from build123d import *

# Parameters (mm, degrees)
SKETCH_1_R      = 1.5
EXTRUDE_2_DEPTH = 24
SKETCH_3_R      = 0.5
EXTRUDE_3_DEPTH = 3.1
FILLET_1_R      = 0.5
SKETCH_4_R      = 3
EXTRUDE_4_DEPTH = 24


with BuildPart() as part:
    # ｽｹｯﾁ1 → ﾎﾞｽ - 押し出し2 (new body)
    with BuildSketch(Plane(origin=(0, 0, 0), x_dir=(1, 0, 0), z_dir=(0, 1, 0))):
        Circle(SKETCH_1_R)
    extrude(amount=EXTRUDE_2_DEPTH)

    # ｽｹｯﾁ3 → ﾎﾞｽ - 押し出し3 (add)
    with BuildSketch(Plane.XZ):
        Circle(SKETCH_3_R)
    extrude(amount=EXTRUDE_3_DEPTH)

    # ﾌｨﾚｯﾄ1
    fillet_1_edges = [part.edges().sort_by_distance(p)[0] for p in [
        (-0.5, -3.1, 0),
    ]]
    fillet(fillet_1_edges, radius=FILLET_1_R)

    # ｽｹｯﾁ4 → ﾎﾞｽ - 押し出し4 (add)
    with BuildSketch(Plane(origin=(0, 24, 0), x_dir=(1, 0, 0), z_dir=(0, 1, 0))):
        Circle(SKETCH_4_R)
    extrude(amount=-EXTRUDE_4_DEPTH)


solid = part.part
Build history of the part. All positions in model axes, mm. A direction names the side the tool comes from. Round coordinates to 2 decimals unless told otherwise and drop trailing zeros. Write each loop counter-clockwise with the first axis right and the second up, starting at its lowest first coordinate (ties: lowest second). Pieces come first, ordered by that corner, then holes. Notation, with made-up numbers: (-14, 2) - (7, 2) arc R19 cw to (7, 15) - close; hole circle Ø11 at (51, -22.5). An arc over 180 degrees is marked (long way). Use CSV: the item, a comma, the result in double quotes.
(1) Band-saw the part on A-A (z = 0). Write the cut outline in (x, y).
Response:
outline,"(-3, 0) - (-0.5, 0) - (-0.5, -2.6) arc R0.5 ccw to (0.5, -2.6) - (0.5, 0) - (3, 0) - (3, 24) - (-3, 24) - close"
(2) Band-saw the part on C-C (y = 16.75). Write the cut outline in (x, z).
Response:
outline,"circle Ø6 at (0, 0)"
(3) 3-axis set-ups, long thin cutter, end or side, ignore diameter. For faces 1 (the cylindrical face through (-3, 12, 0)), 2 (the cylindrical face through (-0.108, -1.282, -0.488)): which of +Z, -Z, +X, -X, +Y, -Y reach the whole face in a straight line?
Response:
face 1,"+Y, -Y"
face 2,"-Y"
(4) Band-saw the part on D-D (x = 2.25). Write the cut outline in (y, z), plus the area to 3 significant figures.
Response:
outline,"(0, -1.98) - (24, -1.98) - (24, 1.98) - (0, 1.98) - close"
area,"95.2 mm²"
(5) Band-saw the part on B-B (x = 0). Write the cut outline in (y, z).
Response:
outline,"(-2.6, -0.5) - (0, -0.5) - (0, -3) - (24, -3) - (24, 3) - (0, 3) - (0, 0.5) - (-2.6, 0.5) arc R0.5 ccw to start"
(6) Pin check, flat tips, straight feed: P1, Ø2, axis at x = -2, z = 0, coming from the -Y side; P2, Ø1.5, axis at x = 2, y = 12, coming from the -Z side. Stop position of each tip, or through.
Response:
P1,"y = 0"
P2,"z = -2.73"
(7) Wall check: line 1 (Y direction, x = 1.75, z = 0.9); line 2 (Z direction, x = -1.2, y = 1.75); line 3 (Z direction, x = -0.85, y = 21.25). Give the ranges that are in metal, low to high.
Response:
line 1,"0 to 24"
line 2,"-2.75 to 2.75"
line 3,"-2.88 to 2.88"
